Geometry: final body of the model. Coordinates: model frame, mm. Face numbers are marked on the shaded views. A direction names the side the tool comes from. Give positions to 0.01 mm unless a question says otherwise; leave off trailing zeros. Order: outer loops, then holes, each group sorted by start corner. A loop starts at its lowest first (then second) coordinate and runs counter-clockwise, first axis right, second up. Notation, with made-up numbers: (23, 34.5) - (67, 34.5) arc R35 cw to (67, 70.5) - close; hole circle Ø3 at (37, 47). An arc over 180 degrees is marked (long way). Put each result on its own line as item: value. Start each with the question number.
1. Ray query, line 1 along Y through (x, z) = (4.5, 17.5); line 2 along Y through (x, z) = (2, 17.25); line 3 along Z through (x, y) = (-10, 6). Return the intervals inside material, ascending. Write a range as from..to.
2. First-contact query: P1, Ø2.5, axis at x = -6, z = 18, coming from the +Y side; P2, Ø4, axis at x = -6.5, z = 18.5, coming from the -Y side; P3, Ø12, axis at y = -3.5, z = 9.5, coming from the +X side. Flat tips, straight axial feed; report the tip coordinate or a pass-through.
3. Section D-D on z = 10. Return the cut outline in (x, y), plus the area to 3 significant figures.
4. Section C-C on y = 0. Return the cut outline in (x, z), plus the area to 3 significant figures.
5. Section A-A on z = 16.5. Return the cut outline in (x, y).
6. Set-up query: the marked faces 1 and 2. Return all of +Z, -Z, +X, -X, +Y, -Y with unobstructed straight access to the full face (end or side cutting, diameter ignored); none if empty.
7. Section B-B on x = 0. Return the cut outline in (y, z), plus the area to 3 significant figures.
from build123d import *

# Parameters (mm, degrees)
ESQUISSE1_R             = 15
BOSS_EXTRU_1_DEPTH      = 20
BOSS_EXTRU_1_DRAFT      = -20
ESQUISSE2_W             = 49.259331118
ESQUISSE2_H             = 5
ENL_V_MAT_EXTRU_1_DEPTH = 5


with BuildPart() as part:
    # Esquisse1 → Boss.-Extru.1 (with draft: the straight prism first)
    with BuildSketch(Plane.XY):
        Circle(ESQUISSE1_R)
    extrude(amount=BOSS_EXTRU_1_DEPTH)
    # Boss.-Extru.1: the draft: its side faces are tilted about the plane it starts from
    boss_extru_1_sides = [part.faces().sort_by_distance(p)[0] for p in [
        (-15, 0, 10),
    ]]
    draft(boss_extru_1_sides, Plane.XY, BOSS_EXTRU_1_DRAFT)

    # Esquisse2 → Enlèv. mat.-Extru.1 (cut)
    with BuildSketch(Plane.XY.offset(20)):
        with Locations((0, -7.5)):
            Rectangle(ESQUISSE2_W, ESQUISSE2_H)
        with Locations((0, 7.5)):
            Rectangle(ESQUISSE2_W, ESQUISSE2_H)
    extrude(amount=-ENL_V_MAT_EXTRU_1_DEPTH, mode=Mode.SUBTRACT)


solid = part.part
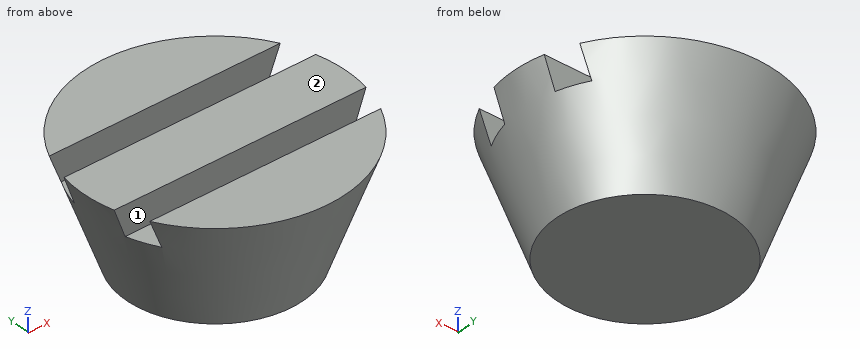
Resolved:
1. line 1: -20.89..-10, -5..5, 10..20.89
1. line 2: -21.18..-10, -5..5, 10..21.18
1. line 3: 0..15
2. P1: y = 21.28
2. P2: y = -21.67
2. P3: x = 20.47
3. outline: circle Ø37.28 at (0, 0)
3. area: 1,090 mm^2
4. outline: (-22.28, 20) - (-15, 0) - (15, 0) - (22.28, 20) - close
4. area: 746 mm^2
5. outline: (-20.4, -5) - (20.4, -5) arc R21.01 ccw to (20.4, 5) - (-20.4, 5) arc R21.01 ccw to start; (-18.47, -10) arc R21.01 ccw to (18.47, -10) - close; (-18.47, 10) - (18.47, 10) arc R21.01 ccw to start
6. face 1: +Z, +X, -X
6. face 2: +Z, +X, -X, +Y, -Y
7. outline: (-22.28, 20) - (-15, 0) - (15, 0) - (22.28, 20) - (10, 20) - (10, 15) - (5, 15) - (5, 20) - (-5, 20) - (-5, 15) - (-10, 15) - (-10, 20) - close
7. area: 696 mm^2
